Geometry check sheet. Reference: the model listing, model coordinates, mm. Face numbers are marked on the shaded views. Give positions to 0.01 mm unless a question says otherwise; leave off trailing zeros. Loops run counter-clockwise (first coordinate to the right, second up) from the corner with the lowest first, then second, coordinate; pieces in that order, holes last.
1. Release check for a two-part mould opening along X. For the marked faces 1 and 2 record: +X half, -X half, draft (parallel to the pull), parting line (faces both ways), or undercut.
2. Cross-section at A-A, the plane z = -4.25. Record the cut outline in (x, y), plus the area to 3 significant figures.
3. Material ranges on L1, parallel to Y at x = 60, z = 0; L2, parallel to X at y = -5.5, z = 2.25; L3, parallel to Y at x = -7, z = 4.25, recorded low to high.
4. Cross-section at B-B, the plane x = 0. Record the cut outline in (y, z), plus the area to 3 significant figures.
5. Cross-section at C-C, the plane y = -2.5. Record the cut outline in (x, z), plus the area to 3 significant figures.
6. Go/stop test with flat-tipped pins: pin 1 Ø10 at (x, y) = (-0.5, -6.5) entering from +Z; pin 2 Ø3 at (x, y) = (27.5, 2) entering from +Z; pin 3 Ø1.3 at (x, z) = (-7, -0.5) entering from -Y; pin 4 Ø4 at (x, z) = (29.5, 0.5) entering from +Y. Record where each tip stops, or that it passes through.
7. Cross-section at D-D, the plane z = -1.25. Record the cut outline in (x, y), plus the area to 3 significant figures.
Autodesk Inventor part; units mm, degrees
ref_plane "YZ Plane" through (0, 0, 0) normal (1, 0, 0) x (0, 1, 0)
ref_plane "XZ Plane" through (0, 0, 0) normal (0, 1, 0) x (-1, 0, 0)
ref_plane "XY Plane" through (0, 0, 0) normal (0, 0, 1) x (1, 0, 0)
sketch "Esboço1" plane through (0, 0, 0) normal (0, 0, 1) x (1, 0, 0)
  circle A0 centre (0, 0) radius 8
  arc A1 (0.8, 11.9733) -> (0.8, -11.9733) centre (0, 0) ccw
  arc A2 (60.5333, -7.9822) -> (60.5333, 7.9822) centre (60, 0) ccw
  circle A3 centre (60, 0) radius 4
  line L0 (0.8, 11.9733) -> (60.5333, 7.9822)
  line L1 (0, 0) -> (60, 0) construction
  line L2 (0.8, -11.9733) -> (60.5333, -7.9822)
  point P0 (-9.6543, 12.6718)
  point P1 (71.6078, 7.2423)
  point P2 (-9.6543, -12.6718)
  point P3 (71.6078, -7.2423)
  dimension "d0" = 16
  dimension "d1" = 24
  dimension "d2" = 16
  dimension "d3" = 8
  dimension "d4" = 60
extrude "Extrusão1" add sketch "Esboço1" along normal mid plane 4
sketch "Esboço2" plane through (0, 0, 0) normal (0, 0, 1) x (1, 0, 0)
  circle A0 centre (0, 0) radius 8
  circle A1 centre (0, 0) radius 12
  circle A2 centre (60, 0) radius 4
  circle A3 centre (60, 0) radius 4
  line L0 (60.5333, 7.9822) -> (0.8, 11.9733)
  circle A4 centre (60, 0) radius 8
extrude "Extrusão2" add sketch "Esboço2" along normal mid plane 12
sketch "Esboço3" plane through (0, 0, 6) normal (0, 0, 1) x (1, 0, 0)
  circle A0 centre (0, 0) radius 8
  line L0 (-8, 0) -> (-6.8, 0)
  line L1 (-6.8, 0) -> (-6.8, 0.6)
  line L2 (-6.8, 0.6) -> (-8, 0.6)
  line L3 (-8, 0.6) -> (-8, 0)
  line L4 (-8, 0) -> (-6.8, 0)
  line L5 (-6.8, 0) -> (-6.8, -0.6)
  line L6 (-6.8, -0.6) -> (-8, -0.6)
  line L7 (-8, -0.6) -> (-8, 0)
  dimension "d9" = 1.2
  dimension "d10" = 0.6
  dimension "d11" = 1.2
  dimension "d12" = 0.6
extrude "Extrusão3" add sketch "Esboço3" against normal blind 12 contours L2 L1 L0 A0 | A0 L3 L2 | L6 L7 A0 | A0 L0 L5 L6
properties part number "Manipulo"
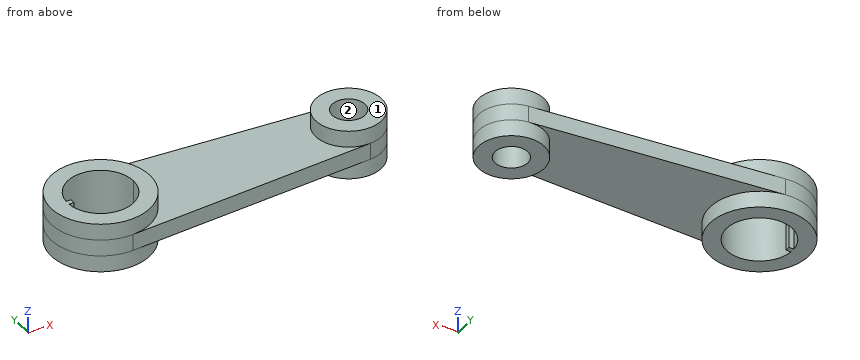
Result:
1. face 1: draft
1. face 2: undercut
2. outline: circle Ø24 at (0, 0); circle Ø16 at (60, 0); hole (-7.98, -0.6) arc R8 ccw (long way) to (-7.98, 0.6) - (-6.8, 0.6) - (-6.8, -0.6) - close; hole circle Ø8 at (60, 0)
2. area: 404 mm2
3. L1: y = -8.02 to -4, 4 to 8.02
3. L2: x = -10.67 to -5.81, 5.81 to 10.67, 54.19 to 65.81
3. L3: y = -9.75 to -3.87, -0.6 to 0.6, 3.87 to 9.75
4. outline: (-12, -6) - (-8, -6) - (-8, 6) - (-12, 6) - (-12, -2) - close; (8, -6) - (12, -6) - (12, -2) - (12, 6) - (8, 6) - close
4. area: 96.0 mm2
5. outline: (-11.74, -6) - (-7.6, -6) - (-7.6, 6) - (-11.74, 6) - (-11.74, -2) - close; (7.6, -6) - (11.74, -6) - (11.74, -2) - (52.4, -2) - (52.4, -6) - (56.88, -6) - (56.88, 6) - (52.4, 6) - (52.4, 2) - (11.74, 2) - (11.74, 6) - (7.6, 6) - close; (63.12, -6) - (67.6, -6) - (67.6, -2) - (67.6, 6) - (63.12, 6) - close
5. area: 369 mm2
6. pin 1: stops at z = 6
6. pin 2: stops at z = 2
6. pin 3: stops at y = -10.18
6. pin 4: stops at y = 10.19
7. outline: (0.8, -11.97) - (60.53, -7.98) arc R8 ccw to (60.53, 7.98) - (0.8, 11.97) arc R12 ccw (long way) to start; hole (-7.98, -0.6) arc R8 ccw (long way) to (-7.98, 0.6) - (-6.8, 0.6) - (-6.8, -0.6) - close; hole circle Ø8 at (60, 0)
7. area: 1,280 mm2
